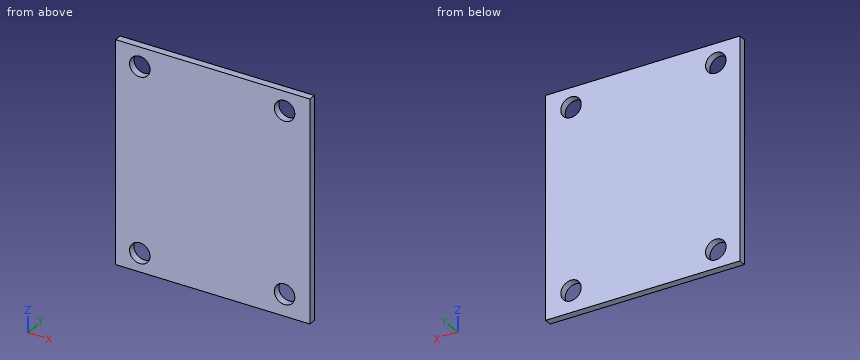
from build123d import *

# Parameters (mm, degrees)
SKETCH1_W                = 32.2
SKETCH1_H                = 36.9
BASE_FLANGE1_DEPTH       = 1.21
M3_CLEARANCE_HOLE1_D     = 3.4
M3_CLEARANCE_HOLE1_DEPTH = 3.34
M3_CLEARANCE_HOLE1_TIP   = 1.021463052


# Sheet-metal steps are written as plain solids
with BuildPart() as part:
    # Sketch1 → Base-Flange1 (new body)
    with BuildSketch(Plane(origin=(0, 0, 0), x_dir=(1, 0, 0), z_dir=(0, 1, 0))):
        Rectangle(SKETCH1_W, SKETCH1_H)
    extrude(amount=-BASE_FLANGE1_DEPTH)

    # M3 Clearance Hole1
    with Locations(Plane(origin=(0, -1.21, 0), x_dir=(-1, 0, 0), z_dir=(0, -1, 0))):
        with Locations((-11.9, -15.248294706), (12.1, -15.248294706), (12.1, 15.370879883), (-11.9, 14.832508941)):
            Hole(M3_CLEARANCE_HOLE1_D / 2, depth=M3_CLEARANCE_HOLE1_DEPTH)
            with Locations((0, 0, -(M3_CLEARANCE_HOLE1_DEPTH + M3_CLEARANCE_HOLE1_TIP / 2))):  # 118° drill point
                Cone(0, M3_CLEARANCE_HOLE1_D / 2, M3_CLEARANCE_HOLE1_TIP, mode=Mode.SUBTRACT)


solid = part.part
CAD build for the part. Positions are in the model's coordinates, mm. Round coordinates to 2 decimals unless told otherwise and drop trailing zeros. Loops run counter-clockwise (first coordinate to the right, second up) from the corner with the lowest first, then second, coordinate; pieces in that order, holes last.
(1) Cut at B-B (y = -0.7). Give the cut face in (x, z).
(2) Cut at C-C (x = 11). Give the cut face in (y, z).
(3) Cut at A-A (x = -12.1). Give the cut face in (y, z).
(4) Drop a flat-ended pin along its axis: pin 1 (2 mm diameter, centred on x = 11.9, z = 15.25, fed in from +Y). Give the stop position or say it passes through.
(5) Wall check: line 1 along Z through (x, y) = (-12, -0.55); line 2 along Z through (x, y) = (11.9, -0.65); line 3 along X through (y, z) = (-0.5, 15). Give the ranges that are in metal, low to high.
Findings below:
1. outline: (-16.1, -18.45) - (16.1, -18.45) - (16.1, 18.45) - (-16.1, 18.45) - close; hole circle Ø3.4 at (-12.1, -15.37); hole circle Ø3.4 at (-12.1, 15.25); hole circle Ø3.4 at (11.9, -14.83); hole circle Ø3.4 at (11.9, 15.25)
2. outline: (-1.21, -18.45) - (0, -18.45) - (0, -16.27) - (-1.21, -16.27) - close; (-1.21, -13.39) - (0, -13.39) - (0, 13.81) - (-1.21, 13.81) - close; (-1.21, 16.69) - (0, 16.69) - (0, 18.45) - (-1.21, 18.45) - close
3. outline: (-1.21, -18.45) - (0, -18.45) - (0, -17.07) - (-1.21, -17.07) - close; (-1.21, -13.67) - (0, -13.67) - (0, 13.55) - (-1.21, 13.55) - close; (-1.21, 16.95) - (0, 16.95) - (0, 18.45) - (-1.21, 18.45) - close
4. pin 1: passes through
5. line 1: z = -18.45 to -17.07, -13.67 to 13.55, 16.95 to 18.45
5. line 2: z = -18.45 to -16.53, -13.13 to 13.55, 16.95 to 18.45
5. line 3: x = -16.1 to -13.78, -10.42 to 10.22, 13.58 to 16.1
